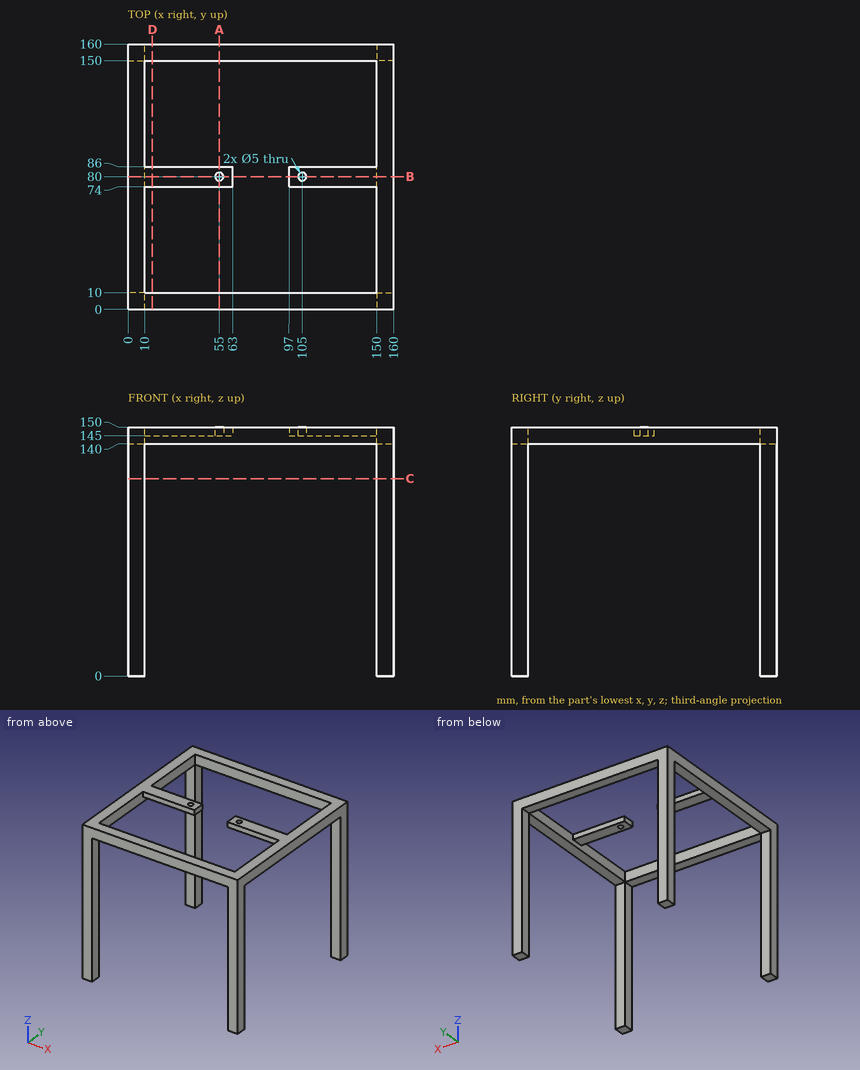
Geometry check sheet. Reference: drawing and pictorial views, mm from the part's lowest x, y, z. Round coordinates to 2 decimals unless told otherwise and drop trailing zeros. Order: outer loops, then holes, each group sorted by start corner. A loop starts at its lowest first (then second) coordinate and runs counter-clockwise, first axis right, second up. Notation, with made-up numbers: (4, -33.5) -> (47, -33.5) arc R34 ccw to (47, 5.5) -> close; hole circle Ø4 at (-12.75, 61.25). An arc over 180 degrees is marked (long way). One line per item, written item: value. Start each with the question number.
Q1. Cross-section at D-D (x = 14.5). Record the boundary of the cut face in (y, z).
Q2. Cross-section at C-C (z = 119). Record the boundary of the cut face in (x, y), and give its area (3 significant figures).
Q3. Cross-section at B-B (y = 80). Record the boundary of the cut face in (x, z), and give its area (3 significant figures).
Q4. Thickness scan on line 1 (X direction, y = 80, z = 148); line 2 (Y direction, x = 55, z = 146.25); line 3 (Y direction, x = 151, z = 20). Record the ranges inside material, lowest first.
Q5. Gauge pin test, flat ends, axial feed: pin 1 Ø5 at (x, y) = (138.5, 81) entering from -Z; pin 2 Ø5 at (x, y) = (84.5, 3) entering from -Z; pin 3 Ø4 at (x, y) = (55, 80) entering from -Z (1 decimal). Record the tip position at first contact, or that the pin passes through.
Q6. Cross-section at A-A (x = 55). Record the boundary of the cut face in (y, z).
Completed:
1. outline: (0, 140) -> (10, 140) -> (10, 150) -> (0, 150) -> close; (74, 145) -> (86, 145) -> (86, 150) -> (74, 150) -> close; (150, 140) -> (160, 140) -> (160, 150) -> (150, 150) -> close
2. outline: (0, 0) -> (10, 0) -> (10, 10) -> (0, 10) -> close; (0, 150) -> (10, 150) -> (10, 160) -> (0, 160) -> close; (150, 0) -> (160, 0) -> (160, 10) -> (150, 10) -> close; (150, 150) -> (160, 150) -> (160, 160) -> (150, 160) -> close
2. area: 400 mm²
3. outline: (0, 140) -> (10, 140) -> (10, 145) -> (52.5, 145) -> (52.5, 150) -> (0, 150) -> close; (57.5, 145) -> (63, 145) -> (63, 150) -> (57.5, 150) -> close; (97, 145) -> (102.5, 145) -> (102.5, 150) -> (97, 150) -> close; (107.5, 145) -> (150, 145) -> (150, 140) -> (160, 140) -> (160, 150) -> (107.5, 150) -> close
3. area: 680 mm²
4. line 1: x = 0 to 52.5, 57.5 to 63, 97 to 102.5, 107.5 to 160
4. line 2: y = 0 to 10, 74 to 77.5, 82.5 to 86, 150 to 160
4. line 3: y = 0 to 10, 150 to 160
5. pin 1: stops at z = 145
5. pin 2: stops at z = 140
5. pin 3: passes through
6. outline: (0, 140) -> (10, 140) -> (10, 150) -> (0, 150) -> close; (74, 145) -> (77.5, 145) -> (77.5, 150) -> (74, 150) -> close; (82.5, 145) -> (86, 145) -> (86, 150) -> (82.5, 150) -> close; (150, 140) -> (160, 140) -> (160, 150) -> (150, 150) -> close
